Design review of the part shown in the three views and the two pictorial views. Dimensions are in mm from the part's minimum x, y and z. A direction names the side the tool comes from. Coordinates: 2 decimals unless noted, no trailing zeros. Loops run counter-clockwise (first coordinate to the right, second up) from the corner with the lowest first, then second, coordinate; pieces in that order, holes last. Notation, with made-up numbers: (68.25, 66.5) - (103.25, 66.5) arc R19 ccw to (103.25, 80.5) - close; hole circle Ø4 at (40, 44.25). An arc over 180 degrees is marked (long way). One line per question, with ' | ' between items.
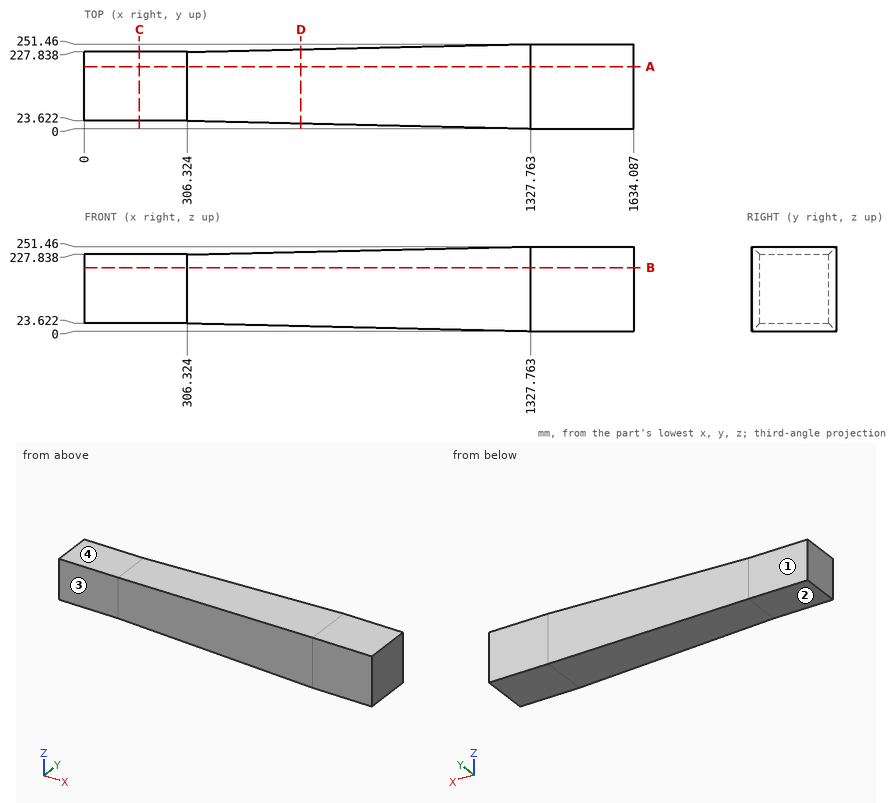
Q1. Take a section at C-C (x = 163.5). Give the boundary of the cut face in (y, z), plus the area to 3 significant figures.
Returned:
outline: (23.62, 23.62) - (227.84, 23.62) - (227.84, 227.84) - (23.62, 227.84) - close | area: 41,700 mm²
Q2. Take a section at D-D (x = 643.5). Give the boundary of the cut face in (y, z), plus the area to 3 significant figures.
Returned:
outline: (15.82, 15.82) - (235.64, 15.82) - (235.64, 235.64) - (15.82, 235.64) - close | area: 48,300 mm²
Q3. To check wall thickness, follow line 1 along Z through (x, y) = (472, 50); line 2 along Z through (x, y) = (351.5, 200); line 3 along Y through (x, z) = (614, 151). State the ranges of each line that lie inside material, in increasing order.
Returned:
line 1: z = 19.79 to 231.67 | line 2: z = 22.58 to 228.88 | line 3: y = 16.51 to 234.95
Q4. Tool access review of the marked faces 1, 2, 3 and 4: name each direction out of +Z, -Z, +X, -X, +Y, -Y from which nothing blocks a thin tool from reaching the whole face with its end or side.
Returned:
face 1: +Z, -Z, -X, +Y | face 2: -Z, -X, +Y, -Y | face 3: +Z, -Z, -X, -Y | face 4: +Z, -X, +Y, -Y
Q5. For pin 1 (10 mm diameter, centred on x = 188.5, z = 107.5, fed in from -Y); pin 2 (5 mm diameter, centred on x = 245.5, y = 123, fed in from +Z); pin 3 (3 mm diameter, centred on x = 1014, z = 202.5, fed in from -Y); pin 4 (3 mm diameter, centred on y = 143, z = 44, fed in from -X), all flat-tipped, find the tip position at first contact; note any pin that passes through.
Returned:
pin 1: stops at y = 23.62 | pin 2: stops at z = 227.84 | pin 3: stops at y = 7.22 | pin 4: stops at x = 0
Q6. Take a section at A-A (y = 184). Give the boundary of the cut face in (x, z), plus the area to 3 significant figures.
Returned:
outline: (0, 23.62) - (306.32, 23.62) - (1327.76, 0) - (1634.09, 0) - (1634.09, 251.46) - (1327.76, 251.46) - (306.32, 227.84) - (0, 227.84) - close | area: 372,000 mm²
